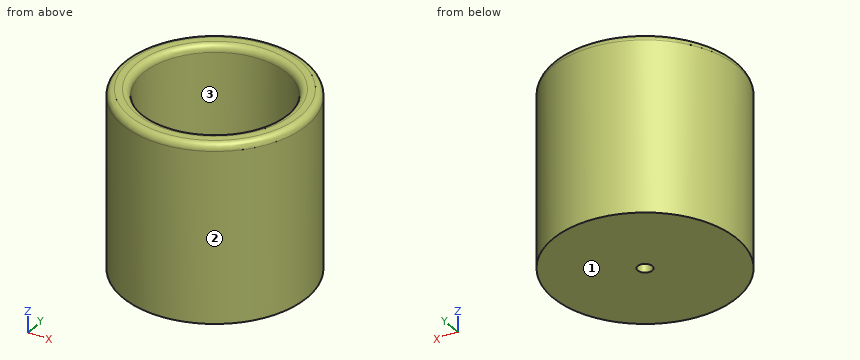
```python
from build123d import *

# Parameters (mm, degrees)
F0_R           = 42.8625
F0_R_2         = 33.3375
F1_DEPTH       = 69.85
F2_R           = 42.8625
F3_DEPTH       = 12.7
F5_D           = 6.7564
F5_CSINK_D     = 13.4874
F5_CSINK_ANGLE = 82
F6_R           = 3.175


with BuildPart() as f1:
    # F0 (on Top) → F1 (new body)
    with BuildSketch(Plane.XY):
        Circle(F0_R)
        Circle(F0_R_2, mode=Mode.SUBTRACT)
    extrude(amount=F1_DEPTH)

    # F2 (on face) → F3 (join)
    with BuildSketch(Plane(origin=(0, 0, 0), x_dir=(1, 0, 0), z_dir=(0, 0, -1))):
        Circle(F2_R)
    extrude(amount=F3_DEPTH)

    # F5 (through all)
    with Locations(Plane.XY):
        with Locations((0, 0)):
            CounterSinkHole(F5_D / 2, F5_CSINK_D / 2, counter_sink_angle=F5_CSINK_ANGLE)

    # F6
    f6_edges = [f1.edges().sort_by_distance(p)[0] for p in [
        (-33.3375, 0, 0),
        (-33.3375, 0, 69.85),
        (-42.8625, 0, 69.85),
    ]]
    fillet(f6_edges, radius=F6_R)


solid = f1.part
```
Work out the finished part from the listing and answer in its coordinate system (mm). Face numbers are marked on the shaded views. Give positions to 0.01 mm unless a question says otherwise; leave off trailing zeros. Order: outer loops, then holes, each group sorted by start corner. A loop starts at its lowest first (then second) coordinate and runs counter-clockwise, first axis right, second up. Notation, with made-up numbers: M 87,-4.5 L 138,-4.5 A19 cw 138,26.5 Z; hole C -7,-27 d8. An arc over 180 degrees is marked long. Return JSON: item names as keys, results as strings.
1) Section C-C, the plane z = 50.5 is taken. Write down the section's boundary in (x, y) (1 decimal), plus the area to 3 significant figures.
Resolved:
{"outline": "C 0,0 d85.7; hole C 0,0 d66.7", "area": "2,280 mm^2"}
2) Straight lines are drawn through the part: line 1 along X through (y, z) = (0, -9.25); line 2 along Y through (x, z) = (0, 48). For each, find the intervals that lie inside material, in ascending order. Write a range as [from, to].
Resolved:
{"line 1": "[-42.86, -3.38], [3.38, 42.86]", "line 2": "[-42.86, -33.34], [33.34, 42.86]"}
3) For a pull along X with two mould halves and no side action, classify the marked faces 1, 2 and 3 as +X half, -X half, draft (parallel to the pull), parting line (faces both ways), or undercut.
Resolved:
{"face 1": "draft", "face 2": "parting line", "face 3": "undercut"}
4) Each of these flat-tipped pins is pushed along its axis until it touches: pin 1 (10 mm diameter, centred on y = -27.5, z = 46, fed in from -X); pin 2 (4 mm diameter, centred on x = 6, z = 19, fed in from +Y); pin 3 (1 mm diameter, centred on x = 8.5, z = 23, fed in from +Y); pin 4 (3 mm diameter, centred on y = 1.5, z = -3.5, fed in from -X). Where does it stop, or does it pass through?
Resolved:
{"pin 1": "x = -36.48", "pin 2": "y = 42.68", "pin 3": "y = 42.11", "pin 4": "x = -42.86"}
